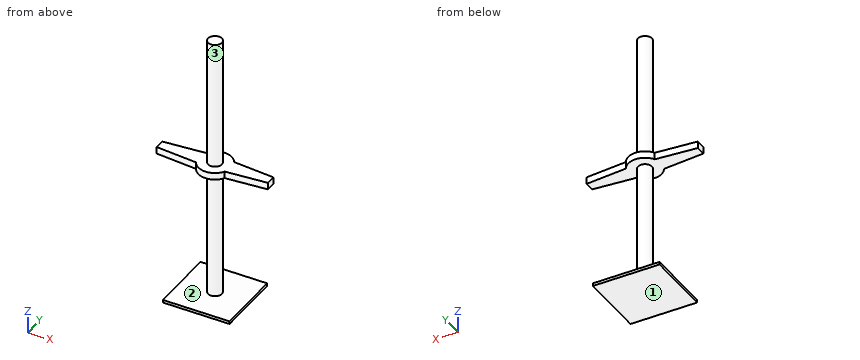
from build123d import *

# Parameters (mm, degrees)
F0_W     = 152.4
F0_H     = 152.4
F1_DEPTH = 6.3754
F2_R     = 15.875
F3_DEPTH = 609.6
F6_DEPTH = 15.875


with BuildPart() as f1:
    # F0 (on Top) → F1 (new body)
    with BuildSketch(Plane.XY):
        Rectangle(F0_W, F0_H)
    extrude(amount=F1_DEPTH)

    # F2 (on face) → F3 (join)
    with BuildSketch(Plane.XY.offset(6.3754)):
        Circle(F2_R)
    extrude(amount=F3_DEPTH)

    # F5 (on offset) → F6 (join)
    with BuildSketch(Plane.XY.offset(304.8)):
        with BuildLine():
            Line((127, 11.1125), (32.995568, 19.05))
            ThreePointArc((32.995568, 19.05), (0, 38.1), (-32.995568, 19.05))
            Line((-32.995568, 19.05), (-127, 11.1125))
            Line((-127, 11.1125), (-127, -11.1125))
            Line((-127, -11.1125), (-32.995568, -19.05))
            ThreePointArc((-32.995568, -19.05), (0, -38.1), (32.995568, -19.05))
            Line((32.995568, -19.05), (127, -11.1125))
            Line((127, -11.1125), (127, 11.1125))
        make_face()
    extrude(amount=F6_DEPTH)


solid = f1.part
Source: CAD feature listing. Evaluate the final solid. Frame: model axes, mm. Face numbers are marked on the shaded views. Give positions to 0.01 mm unless a question says otherwise; leave off trailing zeros. Write each loop counter-clockwise with the first axis right and the second up, starting at its lowest first coordinate (ties: lowest second). Pieces come first, ordered by that corner, then holes. Notation, with made-up numbers: (10, -31.75) - (62, -31.75) arc R21 cw to (62, 3.25) - close; hole circle Ø10 at (64.25, -28). An arc over 180 degrees is marked (long way). Write item = value, one per line. Start each with the question number.
Q1. Cut plane A-A, the plane x = 51. Return loops of the section in (y, z) (3 decimals), then the cut area to 3 significant figures.
Q2. Draft query along Z for the marked faces 1, 2 and 3. Return one class per face: +Z half, -Z half, draft (parallel to the pull), parting line (faces both ways), or undercut.
Q3. Pin query (flat end, axial travel): pin 1 Ø5 at (x, y) = (27.5, 50.5) entering from +Z; pin 2 Ø8 at (y, z) = (16, 447) entering from -X; pin 3 Ø6 at (x, z) = (-13, 75.5) entering from -Y. Return the tip coordinate at first contact, or that it passes through.
Q4. Cut plane D-D, the plane z = 182. Return loops of the section in (x, y) (3 decimals), then the cut area to 3 significant figures.
Q5. Material intervals for probe 1 along Z at (x, y) = (30.5, 18) (3 decimals); probe 2 along Z at (x, y) = (29, 48); probe 3 along Y at (x, z) = (0, 147) (3 decimals), sorted ascending.
Q6. Cut plane B-B, the plane y = 0. Return loops of the section in (x, z) (3 decimals).
Q7. Cut plane C-C, the plane x = 0. Return loops of the section in (y, z) (3 decimals).
Computed values:
q1.outline = (-76.2, 0) - (76.2, 0) - (76.2, 6.375) - (-76.2, 6.375) - close; (-17.53, 304.8) - (17.53, 304.8) - (17.53, 320.675) - (-17.53, 320.675) - close
q1.area = 1,530 mm²
q2.face_1 = -Z half
q2.face_2 = undercut
q2.face_3 = draft
q3.pin_1 = 6.38
q3.pin_2 = -10.39
q3.pin_3 = -12.33
q4.outline = circle Ø31.75 at (0, 0)
q4.area = 792 mm²
q5.probe_1 = 0 to 6.375, 304.8 to 320.675
q5.probe_2 = 0 to 6.38
q5.probe_3 = -15.875 to 15.875
q6.outline = (-127, 304.8) - (-15.875, 304.8) - (-15.875, 6.375) - (-76.2, 6.375) - (-76.2, 0) - (76.2, 0) - (76.2, 6.375) - (15.875, 6.375) - (15.875, 304.8) - (127, 304.8) - (127, 320.675) - (15.875, 320.675) - (15.875, 615.975) - (-15.875, 615.975) - (-15.875, 320.675) - (-127, 320.675) - close
q7.outline = (-76.2, 0) - (76.2, 0) - (76.2, 6.375) - (15.875, 6.375) - (15.875, 304.8) - (38.1, 304.8) - (38.1, 320.675) - (15.875, 320.675) - (15.875, 615.975) - (-15.875, 615.975) - (-15.875, 320.675) - (-38.1, 320.675) - (-38.1, 304.8) - (-15.875, 304.8) - (-15.875, 6.375) - (-76.2, 6.375) - close
